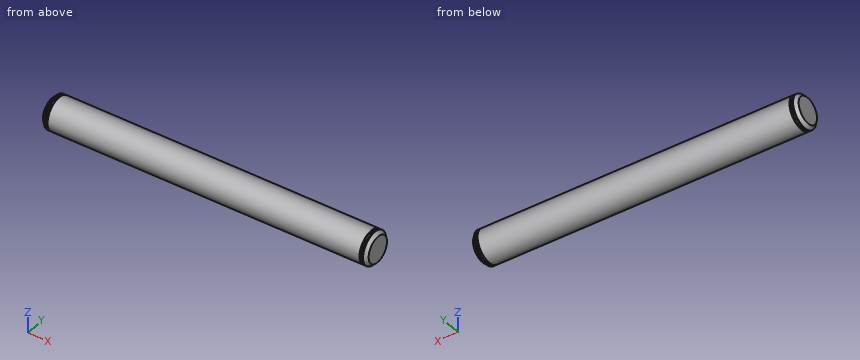
```python
from build123d import *

# Parameters (mm, degrees)
SKETCH2_R           = 6.35
EXTRUDE1_DEPTH      = 63.5
EXTRUDE1_DEPTH_BACK = 63.5
CHAMFER1_SIZE       = 1.27
CUT_EXTRUDE1_START  = 0.5
SKETCH3_R           = 6.35
SKETCH3_R_2         = 5.715
CUT_EXTRUDE1_DEPTH  = 1


with BuildPart() as part:
    # Sketch2 → Extrude1 (new body, two sides)
    with BuildSketch(Plane(origin=(0, 0, 0), x_dir=(0, 0, -1), z_dir=(1, 0, 0))) as extrude1_sk:
        Circle(SKETCH2_R)
    extrude(amount=EXTRUDE1_DEPTH)
    extrude(extrude1_sk.sketch, amount=-EXTRUDE1_DEPTH_BACK)

    # Chamfer1
    chamfer1_edges = [part.edges().sort_by_distance(p)[0] for p in [
        (-63.5, 0, 6.35),
        (63.5, 0, 6.35),
    ]]
    chamfer(chamfer1_edges, length=CHAMFER1_SIZE)

    # Sketch3 → Cut-Extrude1 (cut)
    with BuildSketch(Plane.ZY.offset(60.323942702).offset(CUT_EXTRUDE1_START)):
        Circle(SKETCH3_R)
        Circle(SKETCH3_R_2, mode=Mode.SUBTRACT)
    cut_extrude1 = extrude(amount=CUT_EXTRUDE1_DEPTH, mode=Mode.SUBTRACT)

    # Mirror1: Cut-Extrude1 across plane
    add(cut_extrude1.mirror(Plane(origin=(0, 0, 0), x_dir=(0, 0, 1), z_dir=(1, 0, 0))), mode=Mode.SUBTRACT)


solid = part.part
```
Source: CAD feature listing. Evaluate the final solid. Frame: model axes, mm. Round coordinates to 2 decimals unless told otherwise and drop trailing zeros. Loops run counter-clockwise (first coordinate to the right, second up) from the corner with the lowest first, then second, coordinate; pieces in that order, holes last.
(1) Material intervals for probe 1 along X at (y, z) = (4.25, 4.5); probe 2 along Z at (x, y) = (49, -0.5); probe 3 along Y at (x, z) = (-32, -3.75), sorted ascending.
From the geometry:
probe 1: x = -62.39 to -61.82, -60.82 to 60.82, 61.82 to 62.39
probe 2: z = -6.33 to 6.33
probe 3: y = -5.12 to 5.12
(2) Contact query for flat-ended pins moving along their axis: pin 1 Ø3 at (x, z) = (-4.5, 1.5) entering from -Y; pin 2 Ø2 at (y, z) = (4.5, -4.5) entering from -X; pin 3 Ø1.5 at (x, z) = (-49, -2.5) entering from -Y; pin 4 Ø3 at (x, y) = (48, 2) entering from +Z. Output: stop coordinate, or through.
From the geometry:
pin 1: stops at y = -6.35
pin 2: stops at x = -63.22
pin 3: stops at y = -6.1
pin 4: stops at z = 6.33
(3) Section query A-A (x = -18). Output: boundary loops of the cut face in (y, z), and give its area (3 significant figures).
From the geometry:
outline: circle Ø12.7 at (0, 0)
area: 127 mm2
